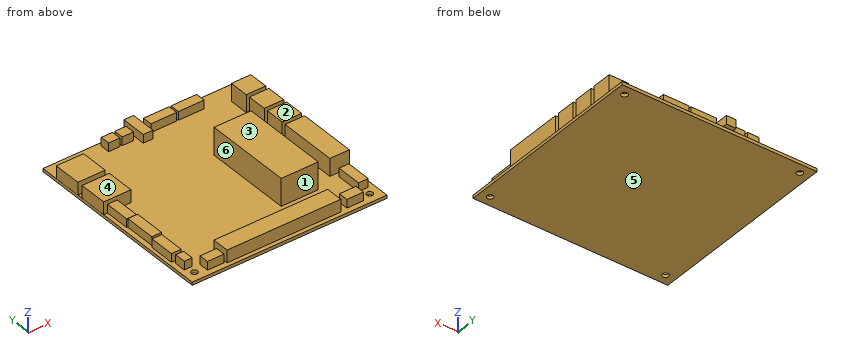
from build123d import *

# Parameters (mm, degrees)
F_100X100_ROTATED_J101_REAR_J801_FRONT_START = 25
SKETCH_1_W                                   = 100
SKETCH_1_H                                   = 100
SKETCH_1_R                                   = 1.6
F_100X100_ROTATED_J101_REAR_J801_FRONT_DEPTH = 1.6
J102_CONNECTOR_ENVELOPE_ROTATED_START        = 26.6
SKETCH_2_W                                   = 10
SKETCH_2_H                                   = 10
J102_CONNECTOR_ENVELOPE_ROTATED_DEPTH        = 9
J201_CONNECTOR_ENVELOPE_ROTATED_START        = 26.6
SKETCH_3_W                                   = 14
SKETCH_3_H                                   = 14.5
J201_CONNECTOR_ENVELOPE_ROTATED_DEPTH        = 6.4
J501_CONNECTOR_ENVELOPE_ROTATED_START        = 26.6
SKETCH_4_W                                   = 14
SKETCH_4_H                                   = 14.5
J501_CONNECTOR_ENVELOPE_ROTATED_DEPTH        = 6.4
J301_CONNECTOR_ENVELOPE_ROTATED_START        = 26.6
SKETCH_5_W                                   = 10
SKETCH_5_H                                   = 10
J301_CONNECTOR_ENVELOPE_ROTATED_DEPTH        = 9
J304_CONNECTOR_ENVELOPE_ROTATED_START        = 26.6
SKETCH_6_W                                   = 10
SKETCH_6_H                                   = 10
J304_CONNECTOR_ENVELOPE_ROTATED_DEPTH        = 9
J302_CONNECTOR_ENVELOPE_ROTATED_START        = 26.6
SKETCH_7_W                                   = 10
SKETCH_7_H                                   = 30
J302_CONNECTOR_ENVELOPE_ROTATED_DEPTH        = 9
J305_CONNECTOR_ENVELOPE_ROTATED_START        = 26.6
SKETCH_8_W                                   = 5.8
SKETCH_8_H                                   = 5
J305_CONNECTOR_ENVELOPE_ROTATED_DEPTH        = 4.35
J306_CONNECTOR_ENVELOPE_ROTATED_START        = 26.6
SKETCH_9_W                                   = 5.8
SKETCH_9_H                                   = 5
J306_CONNECTOR_ENVELOPE_ROTATED_DEPTH        = 4.35
J401_CONNECTOR_ENVELOPE_ROTATED_START        = 26.6
SKETCH_10_W                                  = 5
SKETCH_10_H                                  = 13
J401_CONNECTOR_ENVELOPE_ROTATED_DEPTH        = 4.35
J502_CONNECTOR_ENVELOPE_ROTATED_START        = 26.6
SKETCH_11_W                                  = 5
SKETCH_11_H                                  = 16
J502_CONNECTOR_ENVELOPE_ROTATED_DEPTH        = 4.35
J602_CONNECTOR_ENVELOPE_ROTATED_START        = 26.6
SKETCH_13_W                                  = 5
SKETCH_13_H                                  = 13
J602_CONNECTOR_ENVELOPE_ROTATED_DEPTH        = 4.35
J701_CONNECTOR_ENVELOPE_ROTATED_START        = 26.6
SKETCH_14_W                                  = 5
SKETCH_14_H                                  = 13
J701_CONNECTOR_ENVELOPE_ROTATED_DEPTH        = 4.35
J702_CONNECTOR_ENVELOPE_ROTATED_START        = 26.6
SKETCH_15_W                                  = 13.25
SKETCH_15_H                                  = 5
J702_CONNECTOR_ENVELOPE_ROTATED_DEPTH        = 4.35
J703_CONNECTOR_ENVELOPE_ROTATED_START        = 26.6
SKETCH_16_W                                  = 13.25
SKETCH_16_H                                  = 5
J703_CONNECTOR_ENVELOPE_ROTATED_DEPTH        = 4.35
J704_CONNECTOR_ENVELOPE_ROTATED_START        = 26.6
SKETCH_17_W                                  = 8.5
SKETCH_17_H                                  = 5
J704_CONNECTOR_ENVELOPE_ROTATED_DEPTH        = 4.35
J705_CONNECTOR_ENVELOPE_ROTATED_START        = 26.6
SKETCH_18_W                                  = 5
SKETCH_18_H                                  = 13
J705_CONNECTOR_ENVELOPE_ROTATED_DEPTH        = 4.35
J706_CONNECTOR_ENVELOPE_ROTATED_START        = 26.6
SKETCH_19_W                                  = 8.5
SKETCH_19_H                                  = 5
J706_CONNECTOR_ENVELOPE_ROTATED_DEPTH        = 4.35
J801_CONNECTOR_ENVELOPE_ROTATED_START        = 26.6
SKETCH_20_W                                  = 58.4
SKETCH_20_H                                  = 8.8
J801_CONNECTOR_ENVELOPE_ROTATED_DEPTH        = 6.4
NANO_SOCKET_START                            = 26.6
SKETCH_21_W                                  = 19
SKETCH_21_H                                  = 45
NANO_SOCKET_DEPTH                            = 12.4
NANO_PCB_START                               = 39
SKETCH_22_W                                  = 19
SKETCH_22_H                                  = 45
NANO_PCB_DEPTH                               = 1.6
J601_GH2P_CORRECTED_BODY_REFERENCE_START     = 26.6
SKETCH_23_W                                  = 4.05
SKETCH_23_H                                  = 5.75
J601_GH2P_CORRECTED_BODY_REFERENCE_DEPTH     = 4.35


with BuildPart() as part:
    # 草图1 → 100x100_rotated_J101_rear_J801_front (new body)
    with BuildSketch(Plane.XY.offset(F_100X100_ROTATED_J101_REAR_J801_FRONT_START)):
        with Locations((0, 82)):
            Rectangle(SKETCH_1_W, SKETCH_1_H)
        with Locations((-45, 37)):
            Circle(SKETCH_1_R, mode=Mode.SUBTRACT)
        with Locations((45, 37)):
            Circle(SKETCH_1_R, mode=Mode.SUBTRACT)
        with Locations((45, 127)):
            Circle(SKETCH_1_R, mode=Mode.SUBTRACT)
        with Locations((-45, 127)):
            Circle(SKETCH_1_R, mode=Mode.SUBTRACT)
    extrude(amount=F_100X100_ROTATED_J101_REAR_J801_FRONT_DEPTH)

    # 草图2 → J102_connector_envelope_rotated (add)
    with BuildSketch(Plane.XY.offset(J102_CONNECTOR_ENVELOPE_ROTATED_START)):
        with Locations((44.5045, 117.5895)):
            Rectangle(SKETCH_2_W, SKETCH_2_H)
    extrude(amount=J102_CONNECTOR_ENVELOPE_ROTATED_DEPTH)

    # 草图3 → J201_connector_envelope_rotated (add)
    with BuildSketch(Plane.XY.offset(J201_CONNECTOR_ENVELOPE_ROTATED_START)):
        with Locations((-42.9835, 115.871)):
            Rectangle(SKETCH_3_W, SKETCH_3_H)
    extrude(amount=J201_CONNECTOR_ENVELOPE_ROTATED_DEPTH)

    # 草图4 → J501_connector_envelope_rotated (add)
    with BuildSketch(Plane.XY.offset(J501_CONNECTOR_ENVELOPE_ROTATED_START)):
        with Locations((-42.9835, 98.599)):
            Rectangle(SKETCH_4_W, SKETCH_4_H)
    extrude(amount=J501_CONNECTOR_ENVELOPE_ROTATED_DEPTH)

    # 草图5 → J301_connector_envelope_rotated (add)
    with BuildSketch(Plane.XY.offset(J301_CONNECTOR_ENVELOPE_ROTATED_START)):
        with Locations((44.5045, 93.5225)):
            Rectangle(SKETCH_5_W, SKETCH_5_H)
    extrude(amount=J301_CONNECTOR_ENVELOPE_ROTATED_DEPTH)

    # 草图6 → J304_connector_envelope_rotated (add)
    with BuildSketch(Plane.XY.offset(J304_CONNECTOR_ENVELOPE_ROTATED_START)):
        with Locations((44.5045, 105.5555)):
            Rectangle(SKETCH_6_W, SKETCH_6_H)
    extrude(amount=J304_CONNECTOR_ENVELOPE_ROTATED_DEPTH)

    # 草图7 → J302_connector_envelope_rotated (add)
    with BuildSketch(Plane.XY.offset(J302_CONNECTOR_ENVELOPE_ROTATED_START)):
        with Locations((44.4745, 71.5485)):
            Rectangle(SKETCH_7_W, SKETCH_7_H)
    extrude(amount=J302_CONNECTOR_ENVELOPE_ROTATED_DEPTH)

    # 草图8 → J305_connector_envelope_rotated (add)
    with BuildSketch(Plane.XY.offset(J305_CONNECTOR_ENVELOPE_ROTATED_START)):
        with Locations((-18.7075, 127.555)):
            Rectangle(SKETCH_8_W, SKETCH_8_H)
    extrude(amount=J305_CONNECTOR_ENVELOPE_ROTATED_DEPTH)

    # 草图9 → J306_connector_envelope_rotated (add)
    with BuildSketch(Plane.XY.offset(J306_CONNECTOR_ENVELOPE_ROTATED_START)):
        with Locations((-11.7545, 127.555)):
            Rectangle(SKETCH_9_W, SKETCH_9_H)
    extrude(amount=J306_CONNECTOR_ENVELOPE_ROTATED_DEPTH)

    # 草图10 → J401_connector_envelope_rotated (add)
    with BuildSketch(Plane.XY.offset(J401_CONNECTOR_ENVELOPE_ROTATED_START)):
        with Locations((44.7985, 47.5445)):
            Rectangle(SKETCH_10_W, SKETCH_10_H)
    extrude(amount=J401_CONNECTOR_ENVELOPE_ROTATED_DEPTH)

    # 草图11 → J502_connector_envelope_rotated (add)
    with BuildSketch(Plane.XY.offset(J502_CONNECTOR_ENVELOPE_ROTATED_START)):
        with Locations((-44.972, 70.4055)):
            Rectangle(SKETCH_11_W, SKETCH_11_H)
    extrude(amount=J502_CONNECTOR_ENVELOPE_ROTATED_DEPTH)

    # 草图13 → J602_connector_envelope_rotated (add)
    with BuildSketch(Plane.XY.offset(J602_CONNECTOR_ENVELOPE_ROTATED_START)):
        with Locations((-45.785, 54.6575)):
            Rectangle(SKETCH_13_W, SKETCH_13_H)
    extrude(amount=J602_CONNECTOR_ENVELOPE_ROTATED_DEPTH)

    # 草图14 → J701_connector_envelope_rotated (add)
    with BuildSketch(Plane.XY.offset(J701_CONNECTOR_ENVELOPE_ROTATED_START)):
        with Locations((-45.506, 85.0105)):
            Rectangle(SKETCH_14_W, SKETCH_14_H)
    extrude(amount=J701_CONNECTOR_ENVELOPE_ROTATED_DEPTH)

    # 草图15 → J702_connector_envelope_rotated (add)
    with BuildSketch(Plane.XY.offset(J702_CONNECTOR_ENVELOPE_ROTATED_START)):
        with Locations((6.7595, 127.709)):
            Rectangle(SKETCH_15_W, SKETCH_15_H)
    extrude(amount=J702_CONNECTOR_ENVELOPE_ROTATED_DEPTH)

    # 草图16 → J703_connector_envelope_rotated (add)
    with BuildSketch(Plane.XY.offset(J703_CONNECTOR_ENVELOPE_ROTATED_START)):
        with Locations((20.9175, 127.709)):
            Rectangle(SKETCH_16_W, SKETCH_16_H)
    extrude(amount=J703_CONNECTOR_ENVELOPE_ROTATED_DEPTH)

    # 草图17 → J704_connector_envelope_rotated (add)
    with BuildSketch(Plane.XY.offset(J704_CONNECTOR_ENVELOPE_ROTATED_START)):
        with Locations((-35.7195, 37.359)):
            Rectangle(SKETCH_17_W, SKETCH_17_H)
    extrude(amount=J704_CONNECTOR_ENVELOPE_ROTATED_DEPTH)

    # 草图18 → J705_connector_envelope_rotated (add)
    with BuildSketch(Plane.XY.offset(J705_CONNECTOR_ENVELOPE_ROTATED_START)):
        with Locations((-4.3005, 127.704)):
            Rectangle(SKETCH_18_W, SKETCH_18_H)
    extrude(amount=J705_CONNECTOR_ENVELOPE_ROTATED_DEPTH)

    # 草图19 → J706_connector_envelope_rotated (add)
    with BuildSketch(Plane.XY.offset(J706_CONNECTOR_ENVELOPE_ROTATED_START)):
        with Locations((35.7815, 37.232)):
            Rectangle(SKETCH_19_W, SKETCH_19_H)
    extrude(amount=J706_CONNECTOR_ENVELOPE_ROTATED_DEPTH)

    # 草图20 → J801_connector_envelope_rotated (add)
    with BuildSketch(Plane.XY.offset(J801_CONNECTOR_ENVELOPE_ROTATED_START)):
        with Locations((-1.325, 38.466)):
            Rectangle(SKETCH_20_W, SKETCH_20_H)
    extrude(amount=J801_CONNECTOR_ENVELOPE_ROTATED_DEPTH)

    # 草图21 → Nano_socket (add)
    with BuildSketch(Plane.XY.offset(NANO_SOCKET_START)):
        with Locations((20.5, 74.5)):
            Rectangle(SKETCH_21_W, SKETCH_21_H)
    extrude(amount=NANO_SOCKET_DEPTH)

    # 草图22 → Nano_PCB (add)
    with BuildSketch(Plane.XY.offset(NANO_PCB_START)):
        with Locations((20.5, 74.5)):
            Rectangle(SKETCH_22_W, SKETCH_22_H)
    extrude(amount=NANO_PCB_DEPTH)

    # 草图23 → J601_GH2P_corrected_body_reference (add)
    with BuildSketch(Plane.XY.offset(J601_GH2P_CORRECTED_BODY_REFERENCE_START)):
        with Locations((-45.353, 43.6075)):
            Rectangle(SKETCH_23_W, SKETCH_23_H)
    extrude(amount=J601_GH2P_CORRECTED_BODY_REFERENCE_DEPTH)


solid = part.part
Can you work these out from the model? Positions are in its coordinate system, mm. Face numbers are marked on the shaded views. A direction names the side the tool comes from. Give positions to 0.01 mm unless a question says otherwise; leave off trailing zeros. Order: outer loops, then holes, each group sorted by start corner. A loop starts at its lowest first (then second) coordinate and runs counter-clockwise, first axis right, second up. Notation, with made-up numbers: M -38.5,2.5 L 10.5,2.5 A19 cw 10.5,35.5 Z; hole C 4.25,-18.75 d3. An arc over 180 degrees is marked long. Use a Markdown table: item, result. Add a question column.
Item 1: For the marked faces 1, 2, 3 and 4, which set-ups out of +Z, -Z, +X, -X, +Y, -Y let a thin tool reach every point of the face, with its end or its side?
Item 2: If I drill on L1, parallel to Y at x = -45, z = 25.8; L2, parallel to Y at x = 26, z = 30; L3, parallel to X at y = 64, z = 30, over which ranges is the centre line in solid material (lowest first)? Write a range as [from, to].
Item 3: Suppose I cut it at A-A (y = 37). Count the separate pieces of the cut face and the enclosed holes in it, then the cut area to 3 significant figures.
Item 4: Suppose I cut it at C-C (x = 19.5). List the corners of the cut face in (y, z) for me.
Item 5: Suppose I cut it at D-D (y = 81.5). List the corners of the cut face in (x, z) for me, then the cut area to 3 significant figures.
Item 6: Will these pins go through, and if not, where does the flat tip stop? pin 1 (5 mm diameter, centred on x = 45, z = 29.5, fed in from -Y); pin 2 (2 mm diameter, centred on x = -44.5, z = 28.5, fed in from -Y); pin 3 (6 mm diameter, centred on y = 62, z = 27, fed in from -X); pin 4 (4 mm diameter, centred on x = 36.5, y = 78.5, fed in from +Z).
Item 7: We'd pull the mould along X, two halves only. Please class the marked faces 5 and 6: +X half, -X half, draft (parallel to the pull), parting line (faces both ways), or undercut.
Answer sheet:
| question | item | result |
|---|---|---|
| 1 | face 1 | +Z |
| 1 | face 2 | +Z, +X, +Y, -Y |
| 1 | face 3 | +Z, +X, -X, +Y, -Y |
| 1 | face 4 | +Z, -X, +Y, -Y |
| 2 | L1 | y = [32, 35.4], [38.6, 125.4], [128.6, 132] |
| 2 | L2 | y = [34.07, 42.87], [52, 97], [125.21, 130.21] |
| 2 | L3 | x = [-47.47, -42.47], [11, 30], [39.47, 49.47] |
| 3 | separate pieces | 3 |
| 3 | enclosed holes | 0 |
| 3 | area | 597 mm² |
| 4 | outline | M 32,25 L 132,25 L 132,26.6 L 130.21,26.6 L 130.21,30.95 L 125.21,30.95 L 125.21,26.6 L 97,26.6 L 97,40.6 L 52,40.6 L 52,26.6 L 42.87,26.6 L 42.87,33 L 34.07,33 L 34.07,26.6 L 32,26.6 Z |
| 5 | outline | M -50,25 L 50,25 L 50,26.6 L 49.47,26.6 L 49.47,35.6 L 39.47,35.6 L 39.47,26.6 L 30,26.6 L 30,40.6 L 11,40.6 L 11,26.6 L -43.01,26.6 L -43.01,30.95 L -48.01,30.95 L -48.01,26.6 L -50,26.6 Z |
| 5 | area | 538 mm² |
| 6 | pin 1 | stops at y = 41.04 |
| 6 | pin 2 | stops at y = 40.73 |
| 6 | pin 3 | stops at x = -50 |
| 6 | pin 4 | stops at z = 26.6 |
| 7 | face 5 | draft |
| 7 | face 6 | undercut |
